from build123d import *

# Parameters (mm, degrees)
BASE_DEPTH               = 5
ESBO_O2_R                = 1
FURO_BRACKET_MOTOR_DEPTH = 3
ESBO_O4_W                = 60
ESBO_O4_H                = 70
ENCAIXE_PCB_DEPTH        = 236.334523507
ESBO_O6_R                = 1.5
PARAFUSO_PCB_DEPTH       = 236.334523507
ESBO_O7_R                = 2
ENFORCA_GATO_DEPTH       = 236.334523507
CORTE_EXTRUS_O1_DEPTH    = 10


with BuildPart() as part:
    # Esboço1 → Base (new body)
    with BuildSketch(Plane(origin=(0, 0, 0), x_dir=(1, 0, 0), z_dir=(0, 1, 0))):
        with BuildLine():
            Line((-18.088885989, 17.941465294), (-18.088885989, 19.441465294))
            ThreePointArc((-18.088885989, 19.441465294), (-16.770866504, 22.623445809), (-13.588885989, 23.941465294))
            Line((-13.588885989, 23.941465294), (97.411114011, 23.941465294))
            ThreePointArc((97.411114011, 23.941465294), (100.593094526, 22.623445809), (101.911114011, 19.441465294))
            Line((101.911114011, 19.441465294), (101.911114011, 17.941465294))
            Line((101.911114011, 17.941465294), (101.911114011, -45.8528642))
            ThreePointArc((101.911114011, -45.8528642), (100.781222343, -50.470350333), (97.646878374, -54.044384643))
            Line((97.646878374, -54.044384643), (71.911114011, -72.064760852))
            Line((71.911114011, -72.064760852), (61.911114011, -72.064760852))
            Line((61.911114011, -72.064760852), (54.411114011, -79.564760852))
            Line((54.411114011, -79.564760852), (54.411114011, -162.064760852))
            Line((54.411114011, -162.064760852), (64.411114011, -172.064760852))
            Line((64.411114011, -172.064760852), (91.911114011, -172.064760852))
            Line((91.911114011, -172.064760852), (101.911114011, -182.064760852))
            Line((101.911114011, -182.064760852), (101.911114011, -202.064760852))
            Line((101.911114011, -202.064760852), (91.911114011, -212.064760852))
            Line((91.911114011, -212.064760852), (-8.088885989, -212.064760852))
            Line((-8.088885989, -212.064760852), (-18.088885989, -202.064760852))
            Line((-18.088885989, -202.064760852), (-18.088885989, -182.064760852))
            Line((-18.088885989, -182.064760852), (-8.088885989, -172.064760852))
            Line((-8.088885989, -172.064760852), (19.411114011, -172.064760852))
            Line((19.411114011, -172.064760852), (29.411114011, -162.064760852))
            Line((29.411114011, -162.064760852), (29.411114011, -79.564760852))
            Line((29.411114011, -79.564760852), (21.911114011, -72.064760852))
            Line((21.911114011, -72.064760852), (11.911114011, -72.064760852))
            Line((11.911114011, -72.064760852), (-13.824650353, -54.044384643))
            ThreePointArc((-13.824650353, -54.044384643), (-16.958994321, -50.470350333), (-18.088885989, -45.8528642))
            Line((-18.088885989, -45.8528642), (-18.088885989, 17.941465294))
        make_face()
    extrude(amount=BASE_DEPTH)

    # Esboço2 → Furo Bracket Motor (cut)
    with BuildSketch(Plane(origin=(0, 5, 0), x_dir=(1, 0, 0), z_dir=(0, 1, 0))):
        with Locations(Location((-13.588885989, 19.021465294, 0), (0, 0, 270))):
            Circle(ESBO_O2_R)
        with Locations(Location((-13.588885989, 1.021465294, 0), (0, 0, 270))):
            Circle(ESBO_O2_R)
        with Locations(Location((97.411114011, 1.021465294, 0), (0, 0, 90))):
            Circle(ESBO_O2_R)
        with Locations(Location((97.411114011, 19.021465294, 0), (0, 0, 90))):
            Circle(ESBO_O2_R)
    extrude(amount=-FURO_BRACKET_MOTOR_DEPTH, mode=Mode.SUBTRACT)

    # Esboço4 → Encaixe PCB (cut, through all)
    with BuildSketch(Plane.XZ):
        with Locations((41.911114011, 24.063534706)):
            Rectangle(ESBO_O4_W, ESBO_O4_H)
    extrude(amount=-ENCAIXE_PCB_DEPTH, mode=Mode.SUBTRACT)

    # Esboço6 → Parafuso PCB (cut, through all)
    with BuildSketch(Plane.XZ):
        with Locations(Location((16.911114011, 64.063534706, 0), (0, 0, 270))):
            Circle(ESBO_O6_R)
        with Locations(Location((66.911114011, 64.063534706, 0), (0, 0, 270))):
            Circle(ESBO_O6_R)
        with Locations(Location((66.911114011, -15.936465294, 0), (0, 0, 270))):
            Circle(ESBO_O6_R)
        with Locations(Location((16.911114011, -15.936465294, 0), (0, 0, 270))):
            Circle(ESBO_O6_R)
    extrude(amount=-PARAFUSO_PCB_DEPTH, mode=Mode.SUBTRACT)

    # Esboço7 → Enforca Gato (cut, through all)
    with BuildSketch(Plane.XZ):
        with Locations(Location((33.411114011, 90.814760852, 0), (0, 0, 270))):
            Circle(ESBO_O7_R)
        with Locations(Location((33.411114011, 110.814760852, 0), (0, 0, 270))):
            Circle(ESBO_O7_R)
        with Locations(Location((33.411114011, 130.814760852, 0), (0, 0, 270))):
            Circle(ESBO_O7_R)
        with Locations(Location((33.411114011, 150.814760852, 0), (0, 0, 270))):
            Circle(ESBO_O7_R)
        with Locations(Location((50.411114011, 150.814760852, 0), (0, 0, 90))):
            Circle(ESBO_O7_R)
        with Locations(Location((50.411114011, 130.814760852, 0), (0, 0, 90))):
            Circle(ESBO_O7_R)
        with Locations(Location((50.411114011, 110.814760852, 0), (0, 0, 90))):
            Circle(ESBO_O7_R)
        with Locations(Location((50.411114011, 90.814760852, 0), (0, 0, 90))):
            Circle(ESBO_O7_R)
    extrude(amount=-ENFORCA_GATO_DEPTH, mode=Mode.SUBTRACT)

    # Esboço8 → Corte-extrusão1 (cut)
    with BuildSketch(Plane.XZ):
        with BuildLine():
            ThreePointArc((-11.029836312, 185.987169842), (-10.088885989, 184.189760852), (-9.147935666, 185.987169842))
            ThreePointArc((-9.147935666, 185.987169842), (-3.938885989, 192.064760852), (-9.147935666, 198.142351863))
            ThreePointArc((-9.147935666, 198.142351863), (-10.088885989, 199.939760852), (-11.029836312, 198.142351863))
            ThreePointArc((-11.029836312, 198.142351863), (-16.238885989, 192.064760852), (-11.029836312, 185.987169842))
        make_face()
        with BuildLine():
            ThreePointArc((92.970163688, 185.987169842), (87.761114011, 192.064760852), (92.970163688, 198.142351863))
            ThreePointArc((92.970163688, 198.142351863), (93.911114011, 199.939760852), (94.852064334, 198.142351863))
            ThreePointArc((94.852064334, 198.142351863), (100.061114011, 192.064760852), (94.852064334, 185.987169842))
            ThreePointArc((94.852064334, 185.987169842), (93.911114011, 184.189760852), (92.970163688, 185.987169842))
        make_face()
    extrude(amount=-CORTE_EXTRUS_O1_DEPTH, mode=Mode.SUBTRACT)


solid = part.part
Verification items for the finished model (mm, model axes). A direction names the side the tool comes from. Coordinates: 2 decimals unless noted, no trailing zeros. Order: outer loops, then holes, each group sorted by start corner. A loop starts at its lowest first (then second) coordinate and runs counter-clockwise, first axis right, second up. Notation, with made-up numbers: (78, 44.25) -> (117, 44.25) arc R14 cw to (117, 68.25) -> close; hole circle Ø2 at (58, 54.25). An arc over 180 degrees is marked (long way). Put each result on its own line as item: value. Start each with the question number.
1. Mould release check, pull along Z, two halves, no side actions. Record for faces 1 (the flat face through (41, 2, -10.936)), 2 (the flat face through (67, 2, 72.065)), 3 (the flat face through (41, 2, -23.941)), 4 (the flat face through (-18.089, 2, 14)): released by +Z, released by -Z, zero draft, split by the parting line, or undercut.
2. Access from +Z, -Z, +X, -X, +Y, -Y to the whole of each face (thin tool, end or side, straight path). Record for faces 5 (the flat face through (25.714, 2.465, 75.867)), 6 (the flat face through (43, 0, 92)), 7 (the cylindrical face through (-16.238, 2.465, 192.187)).
3. Cross-section at D-D, the plane z = 168. Record the boundary of the cut face in (x, y), then the cut area to 3 significant figures.
4. Go/stop test with a flat-tipped pin: pin 1 Ø1.8 at (x, z) = (-13.59, -1.02) entering from +Y. Record where the tip stops, or that it passes through.
5. Cross-section at B-B, the plane z = 17. Record the boundary of the cut face in (x, y), then the cut area to 3 significant figures.
6. Cross-section at A-A, the plane x = 45. Record the boundary of the cut face in (y, z).
7. Material ranges on L1, parallel to X at y = 1.7, z = 34.5; L2, parallel to Z at x = 88.5, y = 1.15; L3, parallel to Z at x = 35, y = 0.9, recorded low to high. Write a range as [from, to].
8. Cross-section at C-C, the plane y = 0.8. Count the separate pieces of the cut face and the enclosed holes in it, then the cut area to 4 significant figures.
Computed:
1. face 1: undercut
1. face 2: undercut
1. face 3: released by -Z
1. face 4: zero draft
2. face 5: -X, +Y, -Y
2. face 6: +Z, -Z, +X, -X, -Y
2. face 7: +Y, -Y
3. outline: (23.48, 0) -> (60.35, 0) -> (60.35, 5) -> (23.48, 5) -> close
3. area: 184 mm2
4. pin 1: y = 2
5. outline: (-18.09, 0) -> (11.91, 0) -> (11.91, 5) -> (-18.09, 5) -> close; (71.91, 0) -> (101.91, 0) -> (101.91, 5) -> (71.91, 5) -> close
5. area: 300 mm2
6. outline: (0, -23.94) -> (5, -23.94) -> (5, -10.94) -> (0, -10.94) -> close; (0, 59.06) -> (5, 59.06) -> (5, 212.06) -> (0, 212.06) -> close
7. L1: [-18.09, 11.91], [71.91, 101.91]
7. L2: [-23.94, 60.45], [172.06, 189.14], [194.99, 212.06]
7. L3: [-23.94, -10.94], [59.06, 89.6], [92.03, 109.6], [112.03, 129.6], [132.03, 149.6], [152.03, 212.06]
8. separate pieces: 1
8. enclosed holes: 15
8. area: 13,550 mm2
